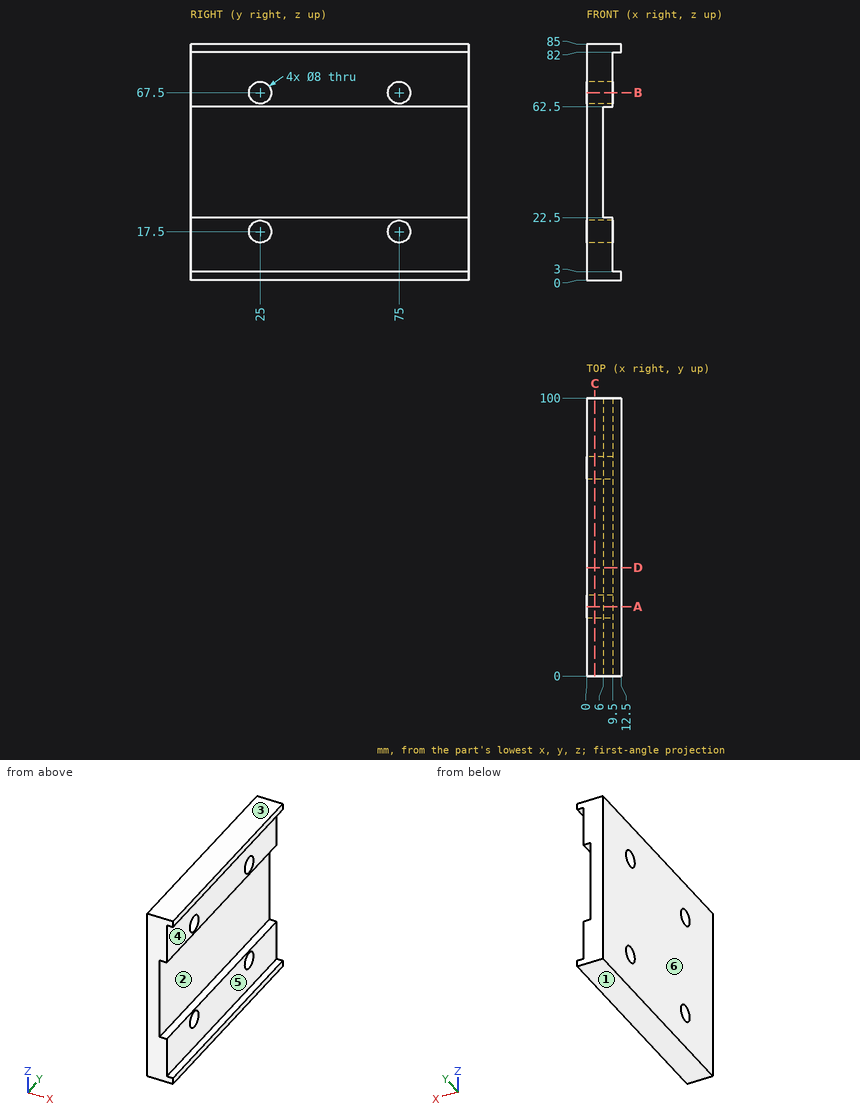
Check sheet for the drawn part. Datum: minimum x, y, z corner. Units: mm. A direction names the side the tool comes from. Round coordinates to 2 decimals unless told otherwise and drop trailing zeros. Order: outer loops, then holes, each group sorted by start corner. A loop starts at its lowest first (then second) coordinate and runs counter-clockwise, first axis right, second up.
(1) Cross-section at C-C, the plane x = 3. Enter the section's corners in (y, z), and give its area (3 significant figures).
(2) Go/stop test with flat-tipped pins: P1, Ø6, axis at y = 35, z = 26, coming from the +X side; P2, Ø13, axis at y = 75, z = 67.5, coming from the +X side. Record where each tip stops, or that it passes through.
(3) Cross-section at A-A, the plane y = 25. Enter the section's corners in (x, z).
(4) Cross-section at B-B, the plane z = 67.5. Enter the section's corners in (x, y).
(5) Cross-section at D-D, the plane y = 39. Enter the section's corners in (x, z).
(6) Scan lines: probe 1 along Z at (x, y) = (2.75, 25); probe 2 along Z at (x, y) = (11.75, 65); probe 3 along Z at (x, y) = (6.5, 15). Record each from-to range of solid material in increasing order.
(7) Draft check along Z on the marked faces 3, 4, 5 and 6. Enter one of: pulls with the +Z half, pulls with the -Z half, needs draft (parallel to the pull), parting line crosses it, or undercut.
(8) Access from +Z, -Z, +X, -X, +Y, -Y to the whole of each face (thin tool, end or side, straight path). Record for the marked faces 1 and 2.
Check sheet entries:
1. outline: (0, 0) - (100, 0) - (100, 85) - (0, 85) - close; hole circle Ø8 at (25, 17.5); hole circle Ø8 at (25, 67.5); hole circle Ø8 at (75, 17.5); hole circle Ø8 at (75, 67.5)
1. area: 8,300 mm2
2. P1: stops at x = 6
2. P2: stops at x = 9.5
3. outline: (0, 0) - (12.5, 0) - (12.5, 3) - (9.5, 3) - (9.5, 13.5) - (0, 13.5) - close; (0, 21.5) - (9.5, 21.5) - (9.5, 22.5) - (6, 22.5) - (6, 62.5) - (9.5, 62.5) - (9.5, 63.5) - (0, 63.5) - close; (0, 71.5) - (9.5, 71.5) - (9.5, 82) - (12.5, 82) - (12.5, 85) - (0, 85) - close
4. outline: (0, 0) - (9.5, 0) - (9.5, 21) - (0, 21) - close; (0, 29) - (9.5, 29) - (9.5, 71) - (0, 71) - close; (0, 79) - (9.5, 79) - (9.5, 100) - (0, 100) - close
5. outline: (0, 0) - (12.5, 0) - (12.5, 3) - (9.5, 3) - (9.5, 22.5) - (6, 22.5) - (6, 62.5) - (9.5, 62.5) - (9.5, 82) - (12.5, 82) - (12.5, 85) - (0, 85) - close
6. probe 1: z = 0 to 13.5, 21.5 to 63.5, 71.5 to 85
6. probe 2: z = 0 to 3, 82 to 85
6. probe 3: z = 0 to 22.5, 62.5 to 85
7. face 3: pulls with the +Z half
7. face 4: undercut
7. face 5: undercut
7. face 6: needs draft
8. face 1: -Z, +X, -X, +Y, -Y
8. face 2: +X, +Y, -Y
